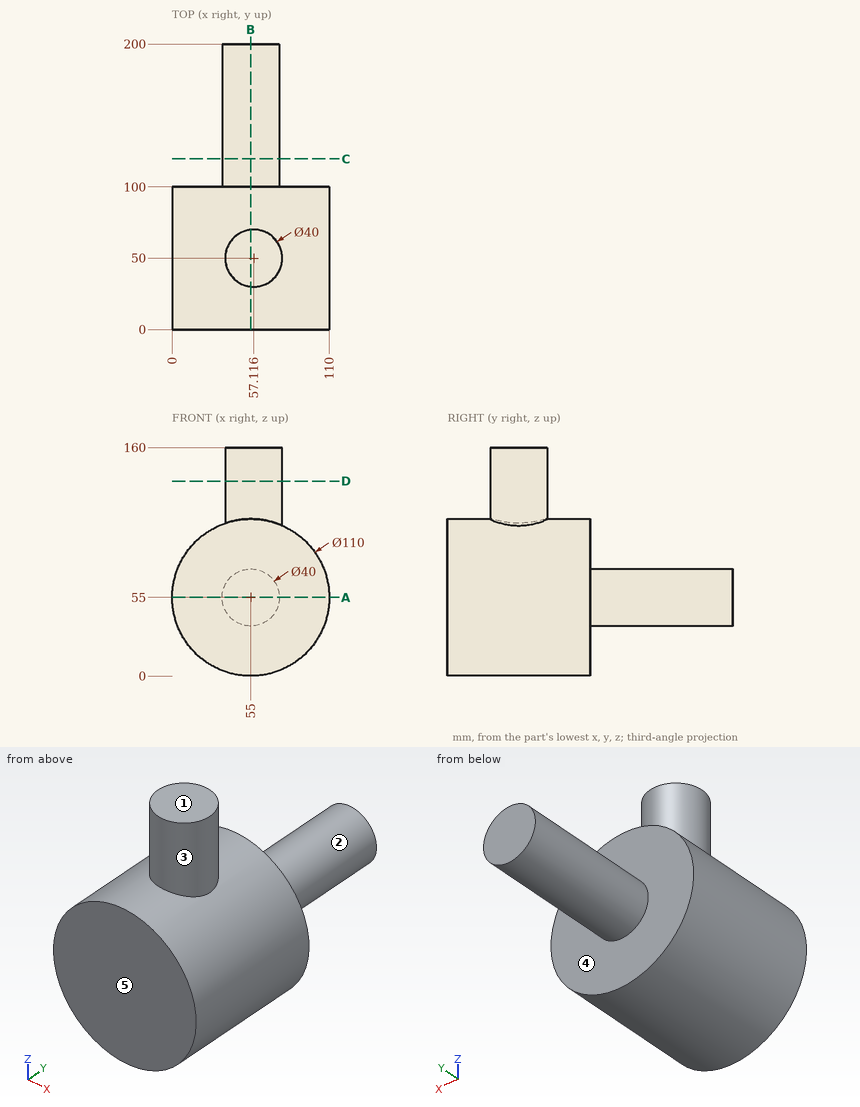
The figure shows three views and two pictorial views of one solid part (mm, origin at its lowest corner). Answer the questions. A direction names the side the tool comes from. Round coordinates to 2 decimals unless told otherwise and drop trailing zeros. Write each loop counter-clockwise with the first axis right and the second up, starting at its lowest first coordinate (ties: lowest second). Pieces come first, ordered by that corner, then holes. Notation, with made-up numbers: (12, 83) - (20, 83) arc R22 ccw to (20, 98) - close; hole circle Ø10 at (-3, -5.5). An arc over 180 degrees is marked (long way). Answer in a Markdown table with one row per item. Add a question column.
1. Find the intervals of material crossed by line 1 along Y through (x, z) = (87, 79); line 2 along Z through (x, y) = (56.5, 16); line 3 along Z through (x, y) = (96, 20), in increasing order. Write a range as from..to.
2. A cutting plane is placed at C-C, the plane y = 119.5. Determine the outline of the cut face in (x, z).
3. For the marked faces 4 and 5, determine the directions among +Z, -Z, +X, -X, +Y, -Y from which every point of the face is accessible in a straight line to the end or side of a thin tool.
4. A cutting plane is placed at D-D, the plane z = 136.5. Determine the outline of the cut face in (x, y).
5. The mould has two halves that part along Z. Classify the marked faces 1, 2 and 3: +Z half, -Z half, draft (parallel to the pull), parting line (faces both ways), or undercut.
6. Given pin 1 (8 mm diameter, centred on x = 83, z = 19.5, fed in from +Y); pin 2 (12 mm diameter, centred on x = 39, y = 100.5, fed in from -Z); pin 3 (1 mm diameter, centred on x = 79, y = 41.5, fed in from -Z); pin 4 (5 mm diameter, centred on x = 56.5, y = 86.5, fed in from -Z), each flat-ended and moving along its own axis, determine where each tip first touches the part or whether it passes through.
7. A cutting plane is placed at A-A, the plane z = 55. Determine the outline of the cut face in (x, y).
8. A cutting plane is placed at B-B, the plane x = 55. Determine the outline of the cut face in (y, z), and give its area (3 significant figures).
Worked out:
| question | item | result |
|---|---|---|
| 1 | line 1 | 0..100 |
| 1 | line 2 | 0.02..109.98 |
| 1 | line 3 | 18.34..91.66 |
| 2 | outline | circle Ø40 at (55, 55) |
| 3 | face 4 | +Y |
| 3 | face 5 | +Z, -Z, +X, -X, -Y |
| 4 | outline | circle Ø40 at (57.12, 50) |
| 5 | face 1 | +Z half |
| 5 | face 2 | parting line |
| 5 | face 3 | draft |
| 6 | pin 1 | y = 100 |
| 6 | pin 2 | z = 0.92 |
| 6 | pin 3 | z = 5.27 |
| 6 | pin 4 | z = 0 |
| 7 | outline | (0, 0) - (110, 0) - (110, 100) - (75, 100) - (75, 200) - (35, 200) - (35, 100) - (0, 100) - close |
| 8 | outline | (0, 0) - (100, 0) - (100, 35) - (200, 35) - (200, 75) - (100, 75) - (100, 110) - (69.89, 110) - (69.89, 160) - (30.11, 160) - (30.11, 110) - (0, 110) - close |
| 8 | area | 17,000 mm^2 |
